```python
from build123d import *

# Parameters (mm, degrees)
F1_DEPTH = 7
F2_R     = 1
F3_DEPTH = 25
F4_SIZE  = 1
F5_R     = 1


with BuildPart() as f1:
    # F0 (on Right) → F1 (new body)
    with BuildSketch(Plane.YZ):
        with BuildLine():
            Line((-39.777774, 0), (-59.777774, 0))
            Line((-59.777774, 0), (-59.777774, -4))
            Line((-59.777774, -4), (-39.777774, -4))
            ThreePointArc((-39.777774, -4), (-30.777774, 5), (-39.777774, 14))
            ThreePointArc((-39.777774, 14), (-41.777774, 12), (-39.777774, 10))
            ThreePointArc((-39.777774, 10), (-34.777774, 5), (-39.777774, 0))
        make_face()
    extrude(amount=F1_DEPTH)

    # F2 (on face) → F3 (cut)
    with BuildSketch(Plane.XY):
        with Locations((3.5, -55.435631)):
            Circle(F2_R)
    extrude(amount=-F3_DEPTH, mode=Mode.SUBTRACT)

    # F4
    f4_edges = [f1.edges().sort_by_distance(p)[0] for p in [
        (2.5, -55.435631, 0),
        (2.5, -55.435631, -4),
    ]]
    chamfer(f4_edges, length=F4_SIZE)

    # F5
    f5_edges = [f1.edges().sort_by_distance(p)[0] for p in [
        (7, -49.777774, 0),
        (7, -34.777774, 5),
        (0, -49.777774, 0),
        (0, -34.777774, 5),
    ]]
    fillet(f5_edges, radius=F5_R)


solid = f1.part
```
Design review of the part built by this model. Coordinates are the model's own, in mm. A direction names the side the tool comes from. Coordinates: 2 decimals unless noted, no trailing zeros. Loops run counter-clockwise (first coordinate to the right, second up) from the corner with the lowest first, then second, coordinate; pieces in that order, holes last. Notation, with made-up numbers: (26.25, 59) -> (48.25, 59) arc R26 ccw to (48.25, 88) -> close; hole circle Ø2 at (57, -33.5). An arc over 180 degrees is marked (long way). Answer as a JSON object with one key per item and string values.
Q1. Tool access review of faces 5 (the flat face through (3, -50, 0)), 6 (the flat face through (3, -59.778, -2)): name each direction out of +Z, -Z, +X, -X, +Y, -Y from which nothing blocks a thin tool from reaching the whole face with its end or side.
Answer block:
{"face 5": "+X, -X, -Y", "face 6": "+Z, -Z, +X, -X, -Y"}
Q2. The part is to be moulded in two halves that separate along Y. For faces 1 (the cylindrical face through (3.46, -34.78, 5.11)), 2 (the cylindrical face through (6.699, -49.638, -3.715)), 3 (the cylindrical face through (3.28, -56.41, -1.99)), 4 (the cylindrical face through (3.46, -30.78, 4.8)), say which applies: +Y half, -Y half, draft (parallel to the pull), parting line (faces both ways), or undercut.
Answer block:
{"face 1": "-Y half", "face 2": "draft", "face 3": "undercut", "face 4": "+Y half"}
Q3. Clearance check with flat-ended pins moving along their axes: pin 1 Ø3 at (x, z) = (1.5, 4.5) entering from -Y; pin 2 Ø2 at (x, z) = (4.5, 7) entering from -Y; pin 3 Ø4 at (x, z) = (6, 11.5) entering from -Y. State where each tip first meets the part, or that it passes through.
Answer block:
{"pin 1": "stops at y = -35.2", "pin 2": "stops at y = -35.78", "pin 3": "stops at y = -41.78"}
Q4. Take a section at C-C on y = -51.25. Give the boundary of the cut face in (x, z).
Answer block:
{"outline": "(0, -3) arc R1 ccw to (1, -4) -> (6, -4) arc R1 ccw to (7, -3) -> (7, -1) arc R1 ccw to (6, 0) -> (1, 0) arc R1 ccw to (0, -1) -> close"}
Q5. Take a section at A-A on x = 3.5. Give the boundary of the cut face in (y, z), plus the area to 3 significant figures.
Answer block:
{"outline": "(-59.78, -4) -> (-57.44, -4) -> (-56.44, -3) -> (-56.44, -1) -> (-57.44, 0) -> (-59.78, 0) -> close; (-54.44, -3) -> (-53.44, -4) -> (-39.78, -4) arc R9 ccw to (-39.78, 14) arc R2 ccw to (-39.78, 10) arc R5 cw to (-39.78, 0) -> (-53.44, 0) -> (-54.44, -1) -> close", "area": "164 mm^2"}
Q6. To check wall thickness, follow L1, parallel to Z at x = 1, y = -56.75; L2, parallel to Y at x = 3.5, z = -1.35; L3, parallel to Z at x = 6.75, y = -36.5. State the ranges of each line that lie inside material, in increasing order.
Answer block:
{"L1": "z = -4 to 0", "L2": "y = -59.78 to -56.44, -54.44 to -33.4", "L3": "z = -3.02 to 0.79, 9.21 to 13.02"}
Q7. Take a section at B-B on z = 5. Give the boundary of the cut face in (x, y), plus the area to 3 significant figures.
Answer block:
{"outline": "(0, -33.78) arc R1 ccw to (1, -34.78) -> (6, -34.78) arc R1 ccw to (7, -33.78) -> (7, -31.78) arc R1 ccw to (6, -30.78) -> (1, -30.78) arc R1 ccw to (0, -31.78) -> close", "area": "27.1 mm^2"}
